Source: CAD feature listing. Evaluate the final solid. Frame: model axes, mm. Give positions to 0.01 mm unless a question says otherwise; leave off trailing zeros. Order: outer loops, then holes, each group sorted by start corner. A loop starts at its lowest first (then second) coordinate and runs counter-clockwise, first axis right, second up. Notation, with made-up numbers: M 5.5,61 L 15.5,61 A24 ccw 15.5,71 Z; hole C 26.5,31.25 d6. An arc over 180 degrees is marked long. Answer in a Markdown table with one row per item. Add a question column.
(1) Pin query (flat end, axial travel): P1, Ø3.5, axis at x = -19.13, y = -46.19, coming from the +Z side; P2, Ø6.5, axis at x = 19.13, y = 46.19, coming from the +Z side; P3, Ø1.5, axis at x = 39, z = 2, coming from the +Y side; P4, Ø1.5, axis at x = 38, z = 2, coming from the +Y side. Return the tip coordinate at first contact, or that it passes through.
(2) Section query A-A, the plane x = 0. Return loops of the section in (y, z), plus the area to 3 significant figures.
(3) Material intervals for line 1 along Y through (x, z) = (0, 1.2); line 2 along Y through (x, z) = (20.5, 2.5); line 3 along X through (y, z) = (-45, 1.55), sorted ascending.
(4) Section query C-C, the plane y = -8.5. Return loops of the section in (x, z), plus the area to 3 significant figures.
(5) Section query B-B, the plane x = -25. Return loops of the section in (y, z).
(6) Section query D-D, the plane z = 1.6. Count the separate pieces of the cut face and the enclosed holes in it, plus the area to 3 significant figures.
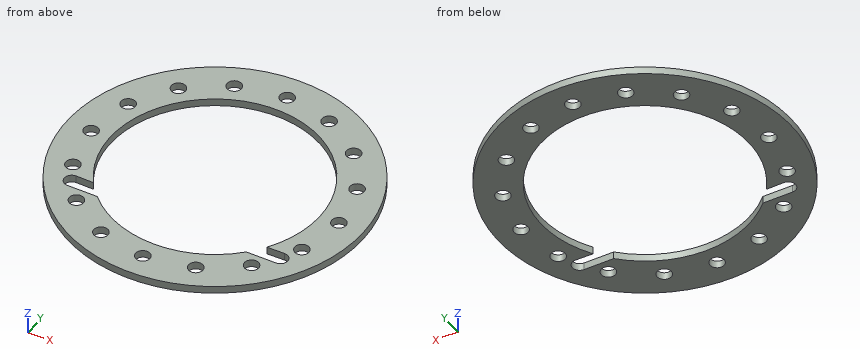
from build123d import *

# Parameters (mm, degrees)
F0_R     = 60
F0_R_2   = 2.9
F1_DEPTH = 3


with BuildPart() as f1:
    # F0 (on Top) → F1 (new body)
    with BuildSketch(Plane.XY):
        Circle(F0_R)
        with Locations((-35.355339, -35.355339)):
            Circle(F0_R_2, mode=Mode.SUBTRACT)
        with Locations((-19.134172, -46.193977)):
            Circle(F0_R_2, mode=Mode.SUBTRACT)
        with Locations((-46.193977, -19.134172)):
            Circle(F0_R_2, mode=Mode.SUBTRACT)
        with Locations((0, -50)):
            Circle(F0_R_2, mode=Mode.SUBTRACT)
        with Locations((19.134172, -46.193977)):
            Circle(F0_R_2, mode=Mode.SUBTRACT)
        with Locations((35.355339, -35.355339)):
            Circle(F0_R_2, mode=Mode.SUBTRACT)
        with Locations((46.193977, -19.134172)):
            Circle(F0_R_2, mode=Mode.SUBTRACT)
        with Locations((-50, 0)):
            Circle(F0_R_2, mode=Mode.SUBTRACT)
        with Locations((-46.193977, 19.134172)):
            Circle(F0_R_2, mode=Mode.SUBTRACT)
        with Locations((-35.355339, 35.355339)):
            Circle(F0_R_2, mode=Mode.SUBTRACT)
        with Locations((-19.134172, 46.193977)):
            Circle(F0_R_2, mode=Mode.SUBTRACT)
        with BuildLine():
            ThreePointArc((-34.982735, -24.134172), (0, 42.5), (34.982735, -24.134172))
            Line((34.982735, -24.134172), (42.083251, -24))
            ThreePointArc((42.083251, -24), (45.083251, -27), (42.083251, -30))
            Line((42.083251, -30), (30.103986, -30))
            ThreePointArc((30.103986, -30), (0, -42.5), (-30.103986, -30))
            Line((-30.103986, -30), (-42.083251, -30))
            ThreePointArc((-42.083251, -30), (-45.083251, -27), (-42.083251, -24))
            Line((-42.083251, -24), (-34.982735, -24.134172))
        make_face(mode=Mode.SUBTRACT)
        with Locations((50, 0)):
            Circle(F0_R_2, mode=Mode.SUBTRACT)
        with Locations((46.193977, 19.134172)):
            Circle(F0_R_2, mode=Mode.SUBTRACT)
        with Locations((0, 50)):
            Circle(F0_R_2, mode=Mode.SUBTRACT)
        with Locations((19.134172, 46.193977)):
            Circle(F0_R_2, mode=Mode.SUBTRACT)
        with Locations((35.355339, 35.355339)):
            Circle(F0_R_2, mode=Mode.SUBTRACT)
    extrude(amount=F1_DEPTH)


solid = f1.part
Values follow:
| question | item | result |
|---|---|---|
| 1 | P1 | passes through |
| 1 | P2 | stops at z = 3 |
| 1 | P3 | stops at y = 46.23 |
| 1 | P4 | stops at y = 47.04 |
| 2 | outline | M -60,0 L -52.9,0 L -52.9,3 L -60,3 Z; M -47.1,0 L -42.5,0 L -42.5,3 L -47.1,3 Z; M 42.5,0 L 47.1,0 L 47.1,3 L 42.5,3 Z; M 52.9,0 L 60,0 L 60,3 L 52.9,3 Z |
| 2 | area | 70.2 mm² |
| 3 | line 1 | y = -60 to -52.9, -47.1 to -42.5, 42.5 to 47.1, 52.9 to 60 |
| 3 | line 2 | y = -56.39 to -48.75, -43.64 to -37.23, 37.23 to 43.64, 48.75 to 56.39 |
| 3 | line 3 | x = -39.69 to -21.78, -16.49 to 16.49, 21.78 to 39.69 |
| 4 | outline | M -59.39,0 L -41.64,0 L -41.64,3 L -59.39,3 Z; M 41.64,0 L 59.39,0 L 59.39,3 L 41.64,3 Z |
| 4 | area | 107 mm² |
| 5 | outline | M -54.54,0 L -34.37,0 L -34.37,3 L -54.54,3 Z; M 34.37,0 L 54.54,0 L 54.54,3 L 34.37,3 Z |
| 6 | separate pieces | 1 |
| 6 | enclosed holes | 17 |
| 6 | area | 5,070 mm² |
